Drawing for the job (mm, zero at the part's lowest x, y, z). A direction names the side the tool comes from. Give positions to 0.01 mm unless a question says otherwise; leave off trailing zeros. Write each loop counter-clockwise with the first axis right and the second up, starting at its lowest first coordinate (ties: lowest second). Pieces come first, ordered by that corner, then holes. Notation, with made-up numbers: (63, 30.25) - (116, 30.25) arc R17 cw to (116, 56.25) - close; hole circle Ø9 at (40, 86). An arc over 180 degrees is marked (long way). Answer as a JSON object with one key per item and string values. Group by question number.
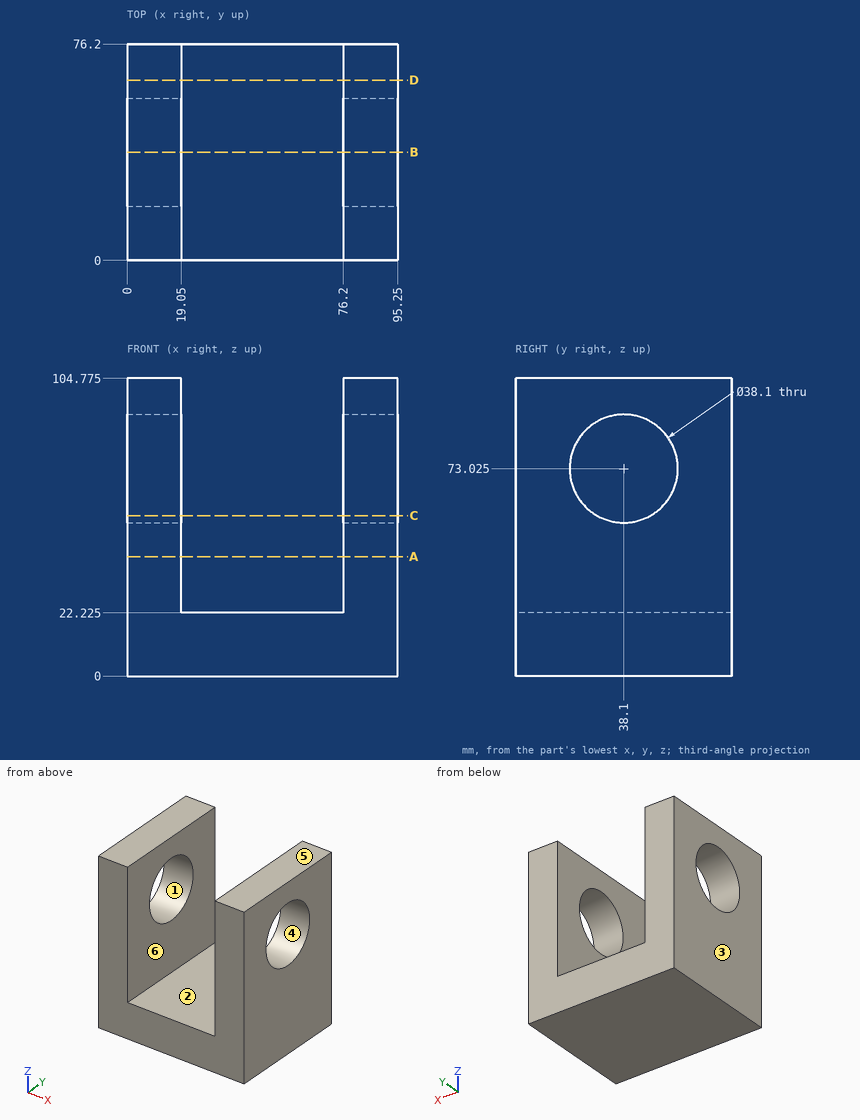
1) Mould opens along Z. For the marked faces 1, 2, 3 and 4 say: pulls with the +Z half, pulls with the -Z half, needs draft (parallel to the pull), parting line crosses it, or undercut.
2) Drop flat-ended pins along their axis: P1, Ø1, axis at x = 49, y = 60.5, coming from the +Z side (3 decimals); P2, Ø23, axis at y = 38.1, z = 73.025, coming from the +X side. Give the stop position or say it passes through.
3) Which spindle directions (+Z, -Z, +X, -X, +Y, -Y) get a long thin tool onto all of the face, cutting with end or side? Do the marked faces 5 and 6. Say none if no direction does.
4) Band-saw the part on A-A (z = 42). List the corners of the cut face in (x, y), plus the area to 3 significant figures.
5) Band-saw the part on D-D (y = 63.5). List the corners of the cut face in (x, z) (3 decimals).
6) Band-saw the part on B-B (y = 38.1). List the corners of the cut face in (x, z) (3 decimals).
7) Probe line 1 (Z direction, x = 88.25, y = 38.1) (3 decimals); line 2 (X direction, y = 19, z = 65.5); line 3 (Z direction, x = 58.5, y = 59) (3 decimals). List the from-to ranges inside material, lowest first.
8) Band-saw the part on C-C (z = 56.5). List the corners of the cut face in (x, y).
Verdict:
{
 "1": {"face 1": "undercut", "face 2": "pulls with the +Z half", "face 3": "needs draft", "face 4": "undercut"},
 "2": {"P1": "z = 22.225", "P2": "through"},
 "3": {"face 5": "+Z, +X, -X, +Y, -Y", "face 6": "+Z, +Y, -Y"},
 "4": {"outline": "(0, 0) - (19.05, 0) - (19.05, 76.2) - (0, 76.2) - close; (76.2, 0) - (95.25, 0) - (95.25, 76.2) - (76.2, 76.2) - close", "area": "2,900 mm2"},
 "5": {"outline": "(0, 0) - (95.25, 0) - (95.25, 104.775) - (76.2, 104.775) - (76.2, 22.225) - (19.05, 22.225) - (19.05, 104.775) - (0, 104.775) - close"},
 "6": {"outline": "(0, 0) - (95.25, 0) - (95.25, 53.975) - (76.2, 53.975) - (76.2, 22.225) - (19.05, 22.225) - (19.05, 53.975) - (0, 53.975) - close; (0, 92.075) - (19.05, 92.075) - (19.05, 104.775) - (0, 104.775) - close; (76.2, 92.075) - (95.25, 92.075) - (95.25, 104.775) - (76.2, 104.775) - close"},
 "7": {"line 1": "0 to 53.975, 92.075 to 104.775", "line 2": "0 to 19.05, 76.2 to 95.25", "line 3": "0 to 22.225"},
 "8": {"outline": "(0, 0) - (19.05, 0) - (19.05, 28.62) - (0, 28.62) - close; (0, 47.58) - (19.05, 47.58) - (19.05, 76.2) - (0, 76.2) - close; (76.2, 0) - (95.25, 0) - (95.25, 28.62) - (76.2, 28.62) - close; (76.2, 47.58) - (95.25, 47.58) - (95.25, 76.2) - (76.2, 76.2) - close"}
}
